Geometry check sheet. Reference: the model listing, model coordinates, mm. Give positions to 0.01 mm unless a question says otherwise; leave off trailing zeros. Write each loop counter-clockwise with the first axis right and the second up, starting at its lowest first coordinate (ties: lowest second). Pieces come first, ordered by that corner, then holes.
(1) Cross-section at A-A (x = 0). Record the boundary of the cut face in (y, z), and give its area (3 significant figures).
(2) Cross-section at B-B (y = -2). Record the boundary of the cut face in (x, z).
(3) Thickness scan on line 1 along X through (y, z) = (-20, -1.35); line 2 along Z through (x, y) = (0, -18.75); line 3 along Z through (x, y) = (-0.3, -4.5). Record the ranges inside material, lowest first.
(4) Mould release check, pull along Z, two halves, no side actions. Record for faces 1 (the flat face through (0, -12, 0)), 2 (the cylindrical face through (0.35, -12.32, -1.94)), 3 (the flat face through (1, 0, -1)): +Z half, -Z half, draft (parallel to the pull), parting line (faces both ways), or undercut.
```python
from build123d import *

# Parameters (mm, degrees)
F1_DEPTH = 25
F2_R     = 0.75
F3_DEPTH = 25


with BuildPart() as f1:
    # F0 (on Front) → F1 (new body)
    with BuildSketch(Plane.XZ):
        with BuildLine():
            Line((1.285368, 0), (-1.314632, 0))
            Line((-1.314632, 0), (-1.314632, -1.3))
            ThreePointArc((-1.314632, -1.3), (-0.014632, -2.6), (1.285368, -1.3))
            Line((1.285368, -1.3), (1.285368, 0))
        make_face()
    extrude(amount=F1_DEPTH)

    # F2 (on Front) → F3 (cut)
    with BuildSketch(Plane.XZ):
        with Locations((0, -1.276303)):
            Circle(F2_R)
    extrude(amount=F3_DEPTH, mode=Mode.SUBTRACT)


solid = f1.part
```
Reply:
1. outline: (-25, -2.6) - (0, -2.6) - (0, -2.03) - (-25, -2.03) - close; (-25, -0.53) - (0, -0.53) - (0, 0) - (-25, 0) - close
1. area: 27.5 mm2
2. outline: (-1.31, -1.3) arc R1.3 ccw to (1.29, -1.3) - (1.29, 0) - (-1.31, 0) - close; hole circle Ø1.5 at (0, -1.28)
3. line 1: x = -1.31 to -0.75, 0.75 to 1.28
3. line 2: z = -2.6 to -2.03, -0.53 to 0
3. line 3: z = -2.57 to -1.96, -0.59 to 0
4. face 1: +Z half
4. face 2: undercut
4. face 3: draft
